Here's the drawing with two shaded views (mm, measured from the low corner). I have some questions. Round coordinates to 2 decimals unless told otherwise and drop trailing zeros. Order: outer loops, then holes, each group sorted by start corner. A loop starts at its lowest first (then second) coordinate and runs counter-clockwise, first axis right, second up.
Q1. If we section it at A-A (x = 53.5): Please give me the cut outline in (y, z), plus the area to 3 significant figures.
Q2. If we section it at B-B (z = 20.25): Please give me the cut outline in (x, y) (3 decimals), plus the area to 3 significant figures.
Q3. If we section it at C-C (y = 47): Please give me the cut outline in (x, z), plus the area to 3 significant figures.
Q4. If I drill on line 1 (Z direction, x = 91, y = 6.5); line 2 (Z direction, x = 13.5, y = 49); line 3 (Y direction, x = 57, z = 22.75), over which ranges is the centre line in solid material (lowest first)?
Q5. Will these pins go through, and if not, where does the flat tip stop? P1, Ø1.5, axis at x = 94, z = 13.5, coming from the -Y side; P2, Ø8, axis at x = 26, z = 20.5, coming from the +Y side; P3, Ø1, axis at x = 80.5, z = 18.5, coming from the -Y side.
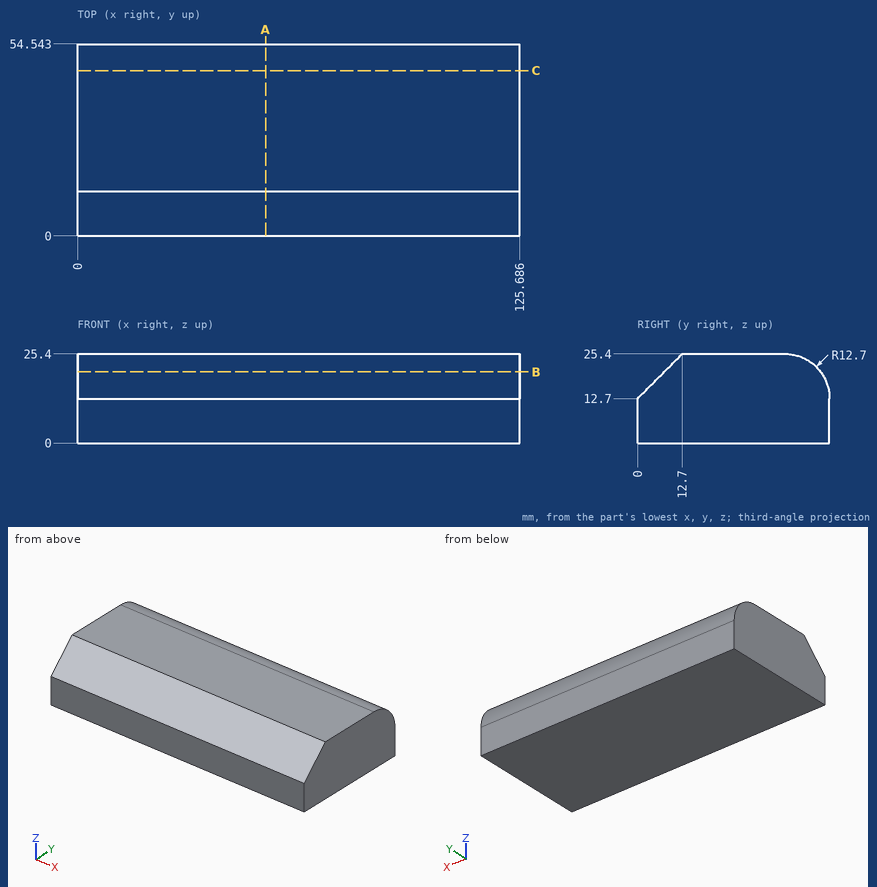
Solution:
1. outline: (0, 0) - (54.54, 0) - (54.54, 12.7) arc R12.7 ccw to (41.84, 25.4) - (12.7, 25.4) - (0, 12.7) - close
1. area: 1,270 mm2
2. outline: (0, 7.55) - (125.686, 7.55) - (125.686, 52.055) - (0, 52.055) - close
2. area: 5,590 mm2
3. outline: (0, 0) - (125.69, 0) - (125.69, 24.31) - (0, 24.31) - close
3. area: 3,050 mm2
4. line 1: z = 0 to 19.2
4. line 2: z = 0 to 23.19
4. line 3: y = 10.05 to 49.61
5. P1: stops at y = 0.05
5. P2: stops at y = 53.96
5. P3: stops at y = 5.3
